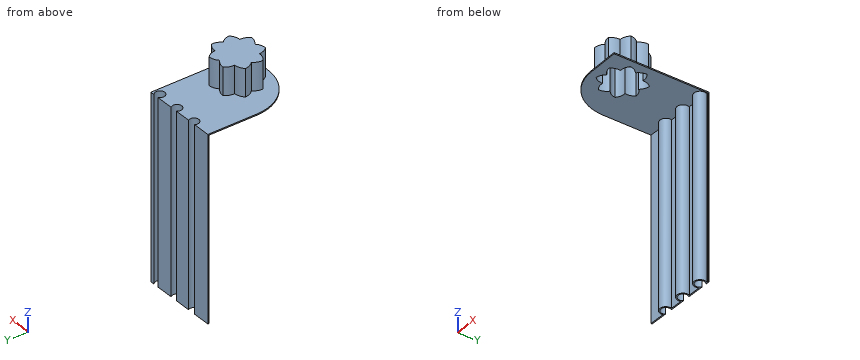
```python
from build123d import *

# Parameters (mm, degrees)
F1_DEPTH      = 228.854
F1_DEPTH_BACK = 170.688
F3_D          = 20.32
F4_R          = 91.9815367264
F5_DEPTH      = 60.198
F6_T          = -2.54


with BuildPart() as f1:
    # F0 (on Top) → F1 (new body, two sides)
    with BuildSketch(Plane.XY) as f1_sk:
        Polygon((-45.7021147013, -62.8560557961), (0, -62.8560557961), (57.0875890553, -62.8560557961), (114.1751781106, -62.8560557961), (114.1751781106, 35.5600006878), (114.1751781106, 126.9761919975), (114.1751781106, 133.9760571718), (114.1751781106, 139.4225805998), (-45.7021147013, 133.9760571718), (-45.7021147013, 35.5600006878), align=None)
    extrude(amount=-F1_DEPTH)
    extrude(f1_sk.sketch, amount=F1_DEPTH_BACK)

    # F3 (through all)
    with Locations(Plane.XY.offset(170.688)):
        with Locations((0, 130.152374506), (50.038, 130.152374506), (100.076, 130.152374506)):
            Hole(F3_D / 2)

    # F4
    f4_edges = [f1.edges().sort_by_distance(p)[0] for p in [
        (-45.702115, -62.856056, -29.083),
    ]]
    fillet(f4_edges, radius=F4_R)

    # F2 (on face) → F5 (join)
    with BuildSketch(Plane.XY.offset(170.688)):
        with BuildLine():
            ThreePointArc((52.7370204776, 37.4581152183), (43.5895428052, 42.9803944735), (33.0250906296, 44.5817270971))
            ThreePointArc((33.0250906296, 44.5817270971), (27.5028113743, 35.4342494247), (25.9014787508, 24.8697972491))
            ThreePointArc((25.9014787508, 24.8697972491), (15.5283941488, 22.3063948652), (6.9258852189, 15.9685122494))
            ThreePointArc((6.9258852189, 15.9685122494), (9.4892876028, 5.5954276475), (15.8271702186, -3.0070812824))
            ThreePointArc((15.8271702186, -3.0070812824), (10.3048909633, -12.1545589549), (8.7035583398, -22.7190111304))
            ThreePointArc((8.7035583398, -22.7190111304), (17.8510360122, -28.2412903857), (28.4154881878, -29.8426230093))
            ThreePointArc((28.4154881878, -29.8426230093), (30.9788905717, -40.2157076112), (37.3167731875, -48.8182165411))
            ThreePointArc((37.3167731875, -48.8182165411), (47.6898577894, -46.2548141572), (56.2923667193, -39.9169315414))
            ThreePointArc((56.2923667193, -39.9169315414), (65.4398443918, -45.4392107967), (76.0042965673, -47.0405434203))
            ThreePointArc((76.0042965673, -47.0405434203), (81.5265758226, -37.8930657478), (83.1279084462, -27.3286135723))
            ThreePointArc((83.1279084462, -27.3286135723), (93.5009930481, -24.7652111884), (102.103501978, -18.4273285726))
            ThreePointArc((102.103501978, -18.4273285726), (99.5400995941, -8.0542439706), (93.2022169783, 0.5482649593))
            ThreePointArc((93.2022169783, 0.5482649593), (98.7244962336, 9.6957426317), (100.3258288572, 20.2601948073))
            ThreePointArc((100.3258288572, 20.2601948073), (91.1783511847, 25.7824740625), (80.6138990092, 27.3838066861))
            ThreePointArc((80.6138990092, 27.3838066861), (78.0504966252, 37.7568912881), (71.7126140095, 46.359400218))
            ThreePointArc((71.7126140095, 46.359400218), (61.3395294075, 43.795997834), (52.7370204776, 37.4581152183))
        make_face()
    extrude(amount=F5_DEPTH)

    # F6
    f6_openings = [f1.faces().sort_by_distance(p)[0] for p in [
        (-18.761346, -35.915287, -29.083),
        (-45.702115, 81.550769, -29.083),
        (37.767676, 39.089228, -228.854),
        (114.175178, 38.283262, -29.083),
        (80.2273, -62.856056, -29.083),
    ]]
    offset(amount=F6_T, openings=f6_openings, kind=Kind.INTERSECTION)


solid = f1.part
```
The listing builds one solid part. Answer for the finished solid, in the listing's coordinates (mm). Round coordinates to 2 decimals unless told otherwise and drop trailing zeros. Loops run counter-clockwise (first coordinate to the right, second up) from the corner with the lowest first, then second, coordinate; pieces in that order, holes last.
Q1. Section D-D, the plane y = 7 is taken. Determine the outline of the cut face in (x, z), then the cut area to 3 significant figures.
Q2. Section C-C, the plane x = -31.5 is taken. Determine the outline of the cut face in (y, z).
Q3. Given pin 1 Ø1.5 at (x, y) = (76.5, 34.5) entering from -Z; pin 2 Ø3 at (x, z) = (15.5, -40) entering from -Y; pin 3 Ø5 at (x, y) = (81.5, 15) entering from -Z; pin 4 Ø16.5 at (x, y) = (100.08, 130.15) entering from -Z (3 decimals), each flat-ended and moving along its own axis, determine where each tip first touches the part or whether it passes through.
Q4. Find the intervals of material crossed by line 1 (X direction, y = 130, z = 139.5); line 2 (Z direction, x = 105, y = 18.5); line 3 (Y direction, x = 0, z = 7), in increasing order.
Q5. Section B-B, the plane z = -86 is taken. Determine the outline of the cut face in (x, y), then the cut area to 3 significant figures.
Completed:
1. outline: (-43, 168.15) - (11.64, 168.15) - (11.64, 228.35) - (94.72, 228.35) - (94.72, 168.15) - (114.18, 168.15) - (114.18, 170.69) - (97.58, 170.69) - (97.58, 230.89) - (8.88, 230.89) - (8.88, 170.69) - (-43, 170.69) - close
1. area: 738 mm2
2. outline: (-19.98, 168.15) - (131.92, 168.15) - (131.92, -228.85) - (134.46, -228.85) - (134.46, 170.69) - (-19.98, 170.69) - close
3. pin 1: stops at z = 168.15
3. pin 2: stops at y = 133.47
3. pin 3: stops at z = 228.35
3. pin 4: passes through
4. line 1: x = -12.7 to -10.16, 10.16 to 12.7, 37.34 to 39.88, 60.2 to 62.74, 87.38 to 89.92, 110.23 to 112.78
4. line 2: z = 168.15 to 170.69
4. line 3: y = 117.45 to 119.99
5. outline: (-45.7, 131.43) - (-12.47, 132.57) arc R12.7 ccw (long way) to (12.28, 133.41) - (38.03, 134.29) arc R12.7 ccw (long way) to (61.74, 135.09) - (88.81, 136.02) arc R12.7 ccw (long way) to (110.92, 136.77) - (114.18, 136.88) - (114.18, 139.42) - (104.88, 139.11) arc R10.16 cw (long way) to (94.68, 138.76) - (57.08, 137.48) arc R10.16 cw (long way) to (42.52, 136.98) - (8.43, 135.82) arc R10.16 cw (long way) to (-8.8, 135.23) - (-45.7, 133.98) - close
5. area: 628 mm2
